Build history of the part. All positions in model axes, mm. Face numbers are marked on the shaded views. Round coordinates to 2 decimals unless told otherwise and drop trailing zeros. Loops run counter-clockwise (first coordinate to the right, second up) from the corner with the lowest first, then second, coordinate; pieces in that order, holes last.
from build123d import *

# Parameters (mm, degrees)
SKETCH1_R                            = 9.0043
SKETCH1_R_2                          = 6.9723
BOSS_EXTRUDE1_DEPTH                  = 19.05
BOSS_EXTRUDE2_DEPTH                  = 49.53
BOSS_EXTRUDE2_DEPTH_BACK             = 6.35
SKETCH2_R                            = 11.0363
SKETCH2_R_2                          = 9.0043
BOSS_EXTRUDE3_REACH                  = 72.334
BOSS_EXTRUDE3_END_RADIUS             = 6.9723
SKETCH3_W                            = 2.54
SKETCH3_H                            = 2.54
BOSS_EXTRUDE3_DIRECTION_2_REACH      = 72.334
BOSS_EXTRUDE3_DIRECTION_2_END_RADIUS = 6.9723


with BuildPart() as part:
    # Sketch1 → Boss-Extrude1 (new body)
    with BuildSketch(Plane(origin=(0, 0, 0), x_dir=(1, 0, 0), z_dir=(0, 1, 0))):
        with Locations(Location((0, 0, 0), (0, 0, 90))):
            Circle(SKETCH1_R)
        with Locations(Location((0, 0, 0), (0, 0, 90))):
            Circle(SKETCH1_R_2, mode=Mode.SUBTRACT)
    extrude(amount=BOSS_EXTRUDE1_DEPTH)

    # Sketch2 → Boss-Extrude2 (add, two sides: drawn at the far end of the back side and taken through both)
    with BuildSketch(Plane(origin=(0, 19.05, 0), x_dir=(1, 0, 0), z_dir=(0, 1, 0)).offset(-BOSS_EXTRUDE2_DEPTH_BACK)):
        with Locations(Location((0, 0, 0), (0, 0, 270))):
            Circle(SKETCH2_R)
        with Locations(Location((0, 0, 0), (0, 0, 90))):
            Circle(SKETCH2_R_2, mode=Mode.SUBTRACT)
    extrude(amount=BOSS_EXTRUDE2_DEPTH + BOSS_EXTRUDE2_DEPTH_BACK)

    # Boss-Extrude3: up to this cylinder (the profile starts inside it)
    boss_extrude3_end = Plane(origin=(0, 1.27, 0), z_dir=(0, -1, 0)) * Cylinder(BOSS_EXTRUDE3_END_RADIUS, 159.6126, mode=Mode.PRIVATE)
    # Sketch3 → Boss-Extrude3 (add, up to the surface)
    with BuildSketch(Plane.XY, mode=Mode.PRIVATE) as boss_extrude3_sk1:
        with Locations((1.27, 1.27)):
            Rectangle(SKETCH3_W, SKETCH3_H)
    boss_extrude3_tool1 = extrude(boss_extrude3_sk1.sketch, amount=BOSS_EXTRUDE3_REACH, mode=Mode.PRIVATE) & boss_extrude3_end
    add(boss_extrude3_tool1.solids().sort_by_distance((1.27, 1.27, 0))[0])

    # Boss-Extrude3 direction 2: up to this cylinder (the profile starts inside it)
    boss_extrude3_direction_2_end = Plane(origin=(0, 1.27, 0), z_dir=(0, -1, 0)) * Cylinder(BOSS_EXTRUDE3_DIRECTION_2_END_RADIUS, 159.6126, mode=Mode.PRIVATE)
    # Sketch3 → Boss-Extrude3 direction 2 (add, up to the surface)
    with BuildSketch(Plane.XY, mode=Mode.PRIVATE) as boss_extrude3_direction_2_sk1:
        with Locations((1.27, 1.27)):
            Rectangle(SKETCH3_W, SKETCH3_H)
    boss_extrude3_direction_2_tool1 = extrude(boss_extrude3_direction_2_sk1.sketch, amount=-BOSS_EXTRUDE3_DIRECTION_2_REACH, mode=Mode.PRIVATE) & boss_extrude3_direction_2_end
    add(boss_extrude3_direction_2_tool1.solids().sort_by_distance((1.27, 1.27, 0))[0])


solid = part.part
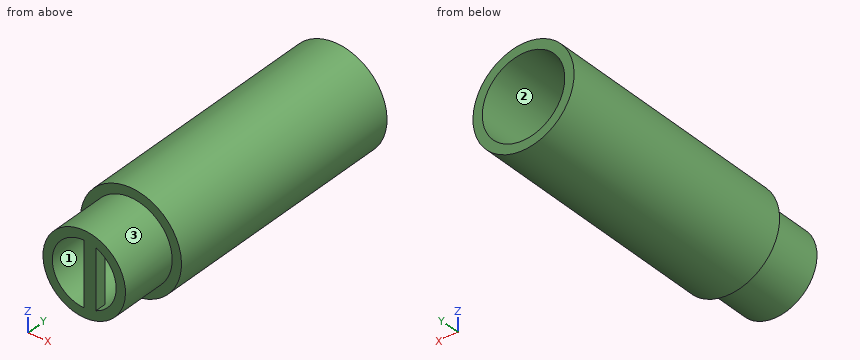
(1) Probe line 1 (X direction, y = 4.5, z = 0); line 2 (X direction, y = 56, z = 0); line 3 (Z direction, x = -4, y = 6). List the from-to ranges inside material, lowest first.
Responses:
line 1: x = -9 to -6.97, 6.97 to 9
line 2: x = -11.04 to -9, 9 to 11.04
line 3: z = -8.07 to -5.71, 5.71 to 8.07
(2) Pin check, flat tips, straight feed: P1, Ø1.3, axis at y = 1.5, z = -3, coming from the -X side; P2, Ø1, axis at y = 30, z = 8, coming from the +X side; P3, Ø1, axis at x = -8, z = -7, coming from the -Y side; P4, Ø4, axis at x = -4.5, z = 0, coming from the +Y side. Stop position of each tip, or through.
Responses:
P1: stops at x = -8.69
P2: stops at x = 8.1
P3: stops at y = 12.7
P4: passes through
(3) Slice it at D-D on z = 3.5. List the corners of the cut face in (x, y), plus the area to 3 significant figures.
Responses:
outline: (-10.47, 12.7) - (-8.3, 12.7) - (-8.3, 0) - (-6.03, 0) - (-6.03, 19.05) - (-8.3, 19.05) - (-8.3, 68.58) - (-10.47, 68.58) - close; (0, 0) - (2.54, 0) - (2.54, 2.54) - (0, 2.54) - close; (6.03, 0) - (8.3, 0) - (8.3, 12.7) - (10.47, 12.7) - (10.47, 68.58) - (8.3, 68.58) - (8.3, 19.05) - (6.03, 19.05) - close
area: 335 mm2
(4) Slice it at B-B on x = 5.75. List the corners of the cut face in (y, z), plus the area to 3 significant figures.
Responses:
outline: (0, -6.93) - (12.7, -6.93) - (12.7, -9.42) - (68.58, -9.42) - (68.58, -6.93) - (19.05, -6.93) - (19.05, -3.94) - (0, -3.94) - close; (0, 3.94) - (19.05, 3.94) - (19.05, 6.93) - (68.58, 6.93) - (68.58, 9.42) - (12.7, 9.42) - (12.7, 6.93) - (0, 6.93) - close
area: 392 mm2
(5) Slice it at A-A on z = 0. List the corners of the cut face in (x, y), plus the area to 3 significant figures.
Responses:
outline: (-11.04, 12.7) - (-9, 12.7) - (-9, 0) - (-6.97, 0) - (-6.97, 19.05) - (-9, 19.05) - (-9, 68.58) - (-11.04, 68.58) - close; (0, 0) - (2.54, 0) - (2.54, 2.54) - (0, 2.54) - close; (6.97, 0) - (9, 0) - (9, 12.7) - (11.04, 12.7) - (11.04, 68.58) - (9, 68.58) - (9, 19.05) - (6.97, 19.05) - close
area: 311 mm2
(6) Pull direction X, two halves, no side cores. Call the marked faces 1, 2 and 3: +X half, -X half, draft (parallel to the pull), parting line (faces both ways), or undercut.
Responses:
face 1: undercut
face 2: undercut
face 3: parting line
(7) Slice it at C-C on y = 38.5. List the corners of the cut face in (x, z), plus the area to 3 significant figures.
Responses:
outline: circle Ø22.07 at (0, 0); hole circle Ø18.01 at (0, 0)
area: 128 mm2
